The listing builds one solid part. Answer for the finished solid, in the listing's coordinates (mm). Face numbers are marked on the shaded views. A direction names the side the tool comes from. Round coordinates to 2 decimals unless told otherwise and drop trailing zeros. Loops run counter-clockwise (first coordinate to the right, second up) from the corner with the lowest first, then second, coordinate; pieces in that order, holes last. Notation, with made-up numbers: (51, 5) -> (61, 5) arc R15 cw to (61, 24) -> close; hole circle Ø9 at (80.5, 67). An arc over 180 degrees is marked (long way). One line per question, with ' | ' between items.
from build123d import *

# Parameters (mm, degrees)
F0_W      = 101.6
F0_H      = 101.6
F1_DEPTH  = 63.5
F2_R      = 38.1
F2_R_2    = 31.75
F3_DEPTH  = 25.4
F3_FACE_R = 31.75
F4_DEPTH  = 63.5


with BuildPart() as f1:
    # F0 (on Top) → F1 (new body)
    with BuildSketch(Plane.XY):
        with Locations((-11.520282, 4.038428)):
            Rectangle(F0_W, F0_H)
    extrude(amount=F1_DEPTH)

    # F2 (on face) → F3 (join)
    with BuildSketch(Plane.XY.offset(63.5)):
        with Locations((-11.520282, 4.038428)):
            Circle(F2_R)
        with Locations((-11.520282, 4.038428)):
            Circle(F2_R_2, mode=Mode.SUBTRACT)
    extrude(amount=F3_DEPTH)

    # F3_face (on face) → F4 (cut)
    with BuildSketch(Plane(origin=(-11.520282, 4.038428, 63.5), x_dir=(1, 0, 0), z_dir=(0, 0, 1))):
        Circle(F3_FACE_R)
    extrude(amount=-F4_DEPTH, mode=Mode.SUBTRACT)


solid = f1.part
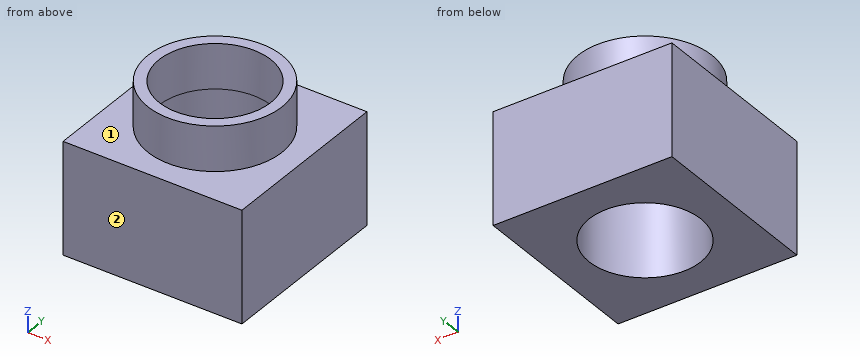
Q1. Given pin 1 Ø1 at (y, z) = (19, 78) entering from +X, flat-ended and moving along its own axis, determine where the tip first touches the part or whether it passes through.
Numbers:
pin 1: x = 23.73
Q2. A cutting plane is placed at D-D on x = -46. Give the vertices of the cut face in (y, z).
Numbers:
outline: (-46.76, 0) -> (54.84, 0) -> (54.84, 63.5) -> (20.25, 63.5) -> (20.25, 88.9) -> (-12.17, 88.9) -> (-12.17, 63.5) -> (-46.76, 63.5) -> close
Q3. A cutting plane is placed at C-C on z = 16. Give the vertices of the cut face in (x, y).
Numbers:
outline: (-62.32, -46.76) -> (39.28, -46.76) -> (39.28, 54.84) -> (-62.32, 54.84) -> close; hole circle Ø63.5 at (-11.52, 4.04)
Q4. Find the intervals of material crossed by line 1 (X direction, y = 30.5, z = 73); line 2 (Y direction, x = 7, z = 33); line 3 (X direction, y = 10.5, z = 13), in increasing order. Write a range as from..to.
Numbers:
line 1: -38.93..-29.07, 6.03..15.89 | line 2: -46.76..-21.75, 29.83..54.84 | line 3: -62.32..-42.61, 19.57..39.28
Q5. A cutting plane is placed at B-B on x = -8.5. Give the vertices of the cut face in (y, z), plus the area to 3 significant figures.
Numbers:
outline: (-46.76, 0) -> (-27.57, 0) -> (-27.57, 88.9) -> (-33.94, 88.9) -> (-33.94, 63.5) -> (-46.76, 63.5) -> close; (35.64, 0) -> (54.84, 0) -> (54.84, 63.5) -> (42.02, 63.5) -> (42.02, 88.9) -> (35.64, 88.9) -> close | area: 2,760 mm^2
Q6. A cutting plane is placed at A-A on y = -25. Give the vertices of the cut face in (x, z), plus the area to 3 significant figures.
Numbers:
outline: (-62.32, 0) -> (-24.36, 0) -> (-24.36, 88.9) -> (-36.19, 88.9) -> (-36.19, 63.5) -> (-62.32, 63.5) -> close; (1.32, 0) -> (39.28, 0) -> (39.28, 63.5) -> (13.15, 63.5) -> (13.15, 88.9) -> (1.32, 88.9) -> close | area: 5,420 mm^2
Q7. For the marked faces 1 and 2, determine the directions among +Z, -Z, +X, -X, +Y, -Y from which every point of the face is accessible in a straight line to the end or side of a thin tool.
Numbers:
face 1: +Z | face 2: +Z, -Z, +X, -X, -Y
